Study the drawing (mm; zero at the part's minimum x, y, z) and answer. A direction names the side the tool comes from. Coordinates: 2 decimals unless noted, no trailing zeros. Loops run counter-clockwise (first coordinate to the right, second up) from the corner with the lowest first, then second, coordinate; pieces in that order, holes last. Notation, with made-up numbers: (8.25, -3.5) - (22.25, -3.5) arc R13 cw to (22.25, 12.5) - close; hole circle Ø1 at (-22, -30). An arc over 180 degrees is marked (long way). Put each result on its own line as item: value.
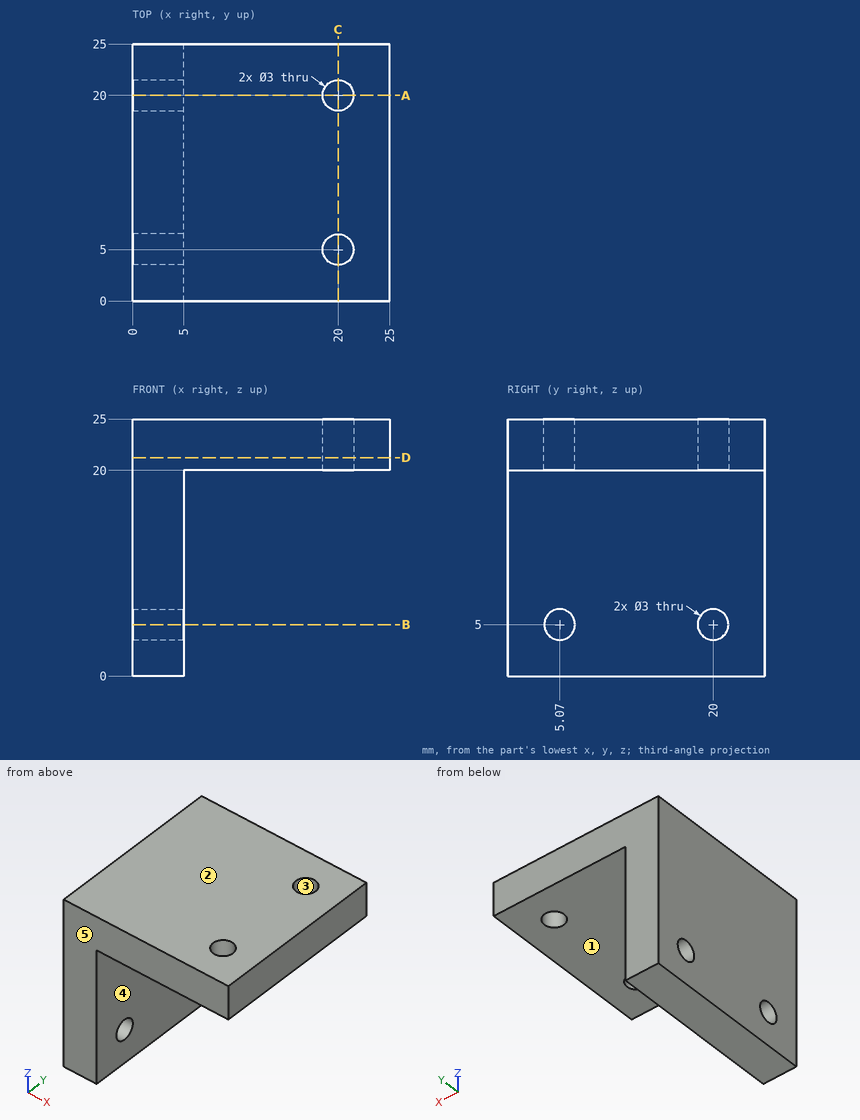
1) For a pull along Y with two mould halves and no side action, classify the marked faces 3, 4 and 5 as pulls with the +Y half, pulls with the -Y half, needs draft (parallel to the pull), parting line crosses it, or undercut.
Found:
face 3: undercut
face 4: needs draft
face 5: pulls with the -Y half
2) Straight lines are drawn through the part: L1, parallel to Y at x = 20, z = 22.85; L2, parallel to Y at x = 3.9, z = 5; L3, parallel to Z at x = 18.5, y = 23. For each, find the intervals that lie inside material, in ascending order. Write a range as [from, to].
Found:
L1: y = [0, 3.5], [6.5, 18.5], [21.5, 25]
L2: y = [0, 3.57], [6.57, 18.5], [21.5, 25]
L3: z = [20, 25]
3) For the marked faces 1 and 2, determine the directions among +Z, -Z, +X, -X, +Y, -Y from which every point of the face is accessible in a straight line to the end or side of a thin tool.
Found:
face 1: -Z, +X, +Y, -Y
face 2: +Z, +X, -X, +Y, -Y
4) The part is cut by section B-B (z = 5). Give the vertices of the cut face in (x, y).
Found:
outline: (0, 0) - (5, 0) - (5, 3.57) - (0, 3.57) - close; (0, 6.57) - (5, 6.57) - (5, 18.5) - (0, 18.5) - close; (0, 21.5) - (5, 21.5) - (5, 25) - (0, 25) - close
5) The part is cut by section C-C (x = 20). Give the vertices of the cut face in (y, z), and give its area (3 significant figures).
Found:
outline: (0, 20) - (3.5, 20) - (3.5, 25) - (0, 25) - close; (6.5, 20) - (18.5, 20) - (18.5, 25) - (6.5, 25) - close; (21.5, 20) - (25, 20) - (25, 25) - (21.5, 25) - close
area: 95.0 mm^2
6) Each of these flat-tipped pins is pushed along its axis until it touches: pin 1 (5 mm diameter, centred on x = 7, y = 18.5, fed in from -Z); pin 2 (12 mm diameter, centred on x = 16, y = 20.5, fed in from -Z); pin 3 (1.8 mm diameter, centred on y = 5.07, z = 5, fed in from -X); pin 4 (10 mm diameter, centred on y = 18.5, z = 13, fed in from +X). Where does it stop, or does it pass through?
Found:
pin 1: stops at z = 0
pin 2: stops at z = 20
pin 3: passes through
pin 4: stops at x = 5
7) The part is cut by section D-D (z = 21.25). Give the vertices of the cut face in (x, y).
Found:
outline: (0, 0) - (25, 0) - (25, 25) - (0, 25) - close; hole circle Ø3 at (20, 5); hole circle Ø3 at (20, 20)
8) The part is cut by section A-A (y = 20). Give the vertices of the cut face in (x, z), and give its area (3 significant figures).
Found:
outline: (0, 0) - (5, 0) - (5, 3.5) - (0, 3.5) - close; (0, 6.5) - (5, 6.5) - (5, 20) - (18.5, 20) - (18.5, 25) - (0, 25) - close; (21.5, 20) - (25, 20) - (25, 25) - (21.5, 25) - close
area: 195 mm^2
